Could you check a few things on this drawing? It's one solid part, dimensions in mm from its lowest x, y, z. Round coordinates to 2 decimals unless told otherwise and drop trailing zeros. Write each loop counter-clockwise with the first axis right and the second up, starting at its lowest first coordinate (ties: lowest second). Pieces come first, ordered by that corner, then holes. Notation, with made-up numbers: (-31.75, 81) -> (-2.75, 81) arc R11 ccw to (-2.75, 101) -> close; hole circle Ø3 at (89.5, 38.25). An arc over 180 degrees is marked (long way). Answer in a Markdown table with one row per item. Add a question column.
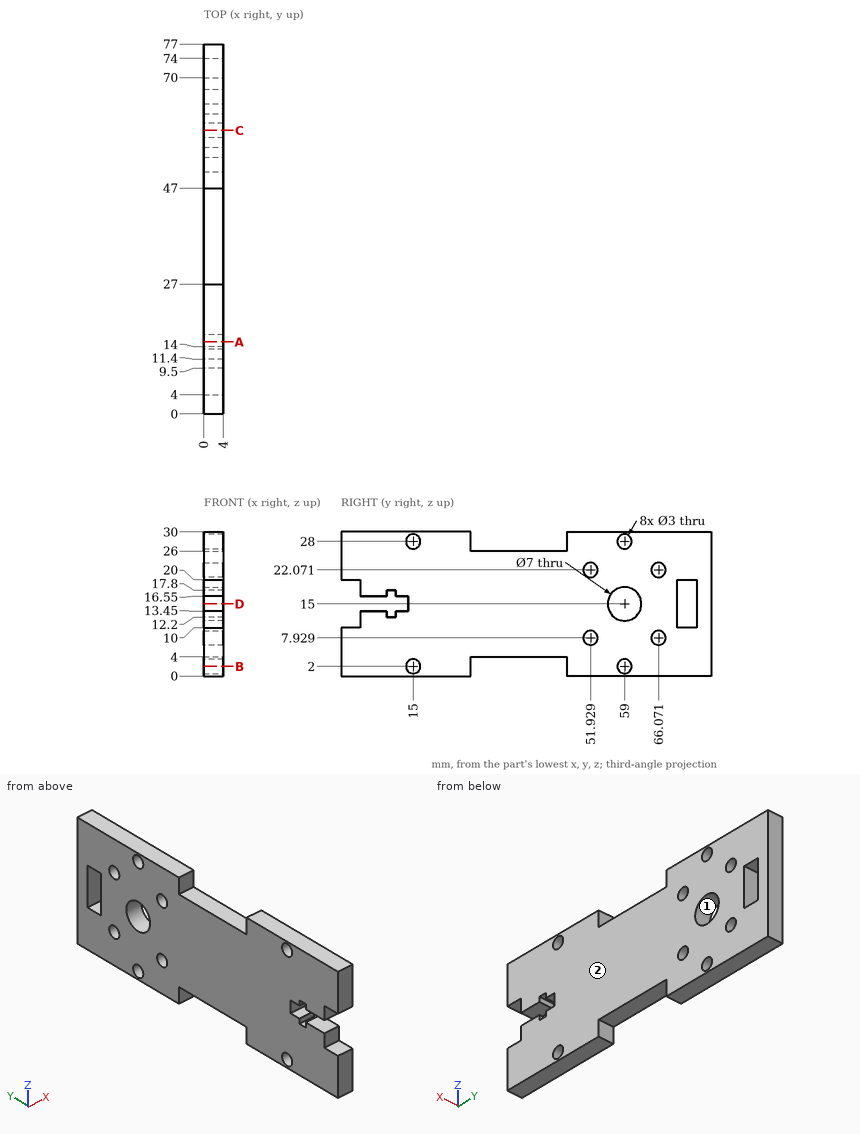
(1) Suppose I cut it at D-D, the plane z = 15. Please give me the cut outline in (x, y).
(2) Suppose I cut it at A-A, the plane y = 15. Please give me the cut outline in (x, z), then the cut area to 3 significant figures.
(3) For P1, Ø1, axis at x = 1, y = 45, coming from the -Z side; P2, Ø0.6, axis at x = 2.5, z = 17, coming from the -Y side, each with a flat end and sliding along its axis, tell me the tip position at first contact or that it passes through.
(4) Suppose I cut it at B-B, the plane z = 2. Please give me the cut outline in (x, y).
(5) Suppose I cut it at C-C, the plane y = 59. Please give me the cut outline in (x, z).
(6) I need wall thicknesses on L1, parallel to Y at x = 3.1, z = 2; L2, parallel to Y at x = 2.4, z = 16.5; L3, parallel to Y at x = 0.7, z = 1.5. Which ranges of each line are inside material? Lowest first, please.
(7) If we mould it in two halves opening along Z, with no side actions, what happens to the marked faces 1 and 2? For each: pulls with the +Z half, pulls with the -Z half, needs draft (parallel to the pull), parting line crosses it, or undercut.
Response:
| question | item | result |
|---|---|---|
| 1 | outline | (0, 14) -> (4, 14) -> (4, 55.5) -> (0, 55.5) -> close; (0, 62.5) -> (4, 62.5) -> (4, 70) -> (0, 70) -> close; (0, 74) -> (4, 74) -> (4, 77) -> (0, 77) -> close |
| 2 | outline | (0, 0) -> (4, 0) -> (4, 0.5) -> (0, 0.5) -> close; (0, 3.5) -> (4, 3.5) -> (4, 26.5) -> (0, 26.5) -> close; (0, 29.5) -> (4, 29.5) -> (4, 30) -> (0, 30) -> close |
| 2 | area | 96.0 mm² |
| 3 | P1 | z = 4 |
| 3 | P2 | y = 4 |
| 4 | outline | (0, 0) -> (4, 0) -> (4, 13.5) -> (0, 13.5) -> close; (0, 16.5) -> (4, 16.5) -> (4, 27) -> (0, 27) -> close; (0, 47) -> (4, 47) -> (4, 57.5) -> (0, 57.5) -> close; (0, 60.5) -> (4, 60.5) -> (4, 77) -> (0, 77) -> close |
| 5 | outline | (0, 0) -> (4, 0) -> (4, 0.5) -> (0, 0.5) -> close; (0, 3.5) -> (4, 3.5) -> (4, 11.5) -> (0, 11.5) -> close; (0, 18.5) -> (4, 18.5) -> (4, 26.5) -> (0, 26.5) -> close; (0, 29.5) -> (4, 29.5) -> (4, 30) -> (0, 30) -> close |
| 6 | L1 | 0 to 13.5, 16.5 to 27, 47 to 57.5, 60.5 to 77 |
| 6 | L2 | 14 to 55.84, 62.16 to 70, 74 to 77 |
| 6 | L3 | 0 to 13.59, 16.41 to 27, 47 to 57.59, 60.41 to 77 |
| 7 | face 1 | undercut |
| 7 | face 2 | needs draft |
